```python
from build123d import *

# Parameters (mm, degrees)
SKETCH1_W           = 10
SKETCH1_H           = 27
BOSS_EXTRUDE1_DEPTH = 10
SKETCH2_R           = 2.5
CUT_EXTRUDE1_DEPTH  = 10
SKETCH3_W           = 4.7
SKETCH3_H           = 4.7
BOSS_EXTRUDE2_DEPTH = 40
SKETCH4_W           = 2
SKETCH4_H           = 62
CUT_EXTRUDE3_DEPTH  = 3
FILLET1_R           = 4
SKETCH5_R           = 3
CUT_EXTRUDE4_DEPTH  = 3
CUT_EXTRUDE5_DEPTH  = 3


with BuildPart() as part:
    # Sketch1 → Boss-Extrude1 (new body)
    with BuildSketch(Plane(origin=(0, 0, 0), x_dir=(1, 0, 0), z_dir=(0, 1, 0))):
        with Locations((0.146426278, 10.467599094)):
            Rectangle(SKETCH1_W, SKETCH1_H)
    extrude(amount=BOSS_EXTRUDE1_DEPTH)

    # Sketch2 → Cut-Extrude1 (cut)
    with BuildSketch(Plane(origin=(0, 10, 0), x_dir=(1, 0, 0), z_dir=(0, 1, 0))):
        with Locations(Location((0.146426278, 18.467599094, 0), (0, 0, 270))):
            Circle(SKETCH2_R)
        with Locations(Location((0.146426278, 10.467599094, 0), (0, 0, 270))):
            Circle(SKETCH2_R)
        with Locations(Location((0.146426278, 2.467599094, 0), (0, 0, 270))):
            Circle(SKETCH2_R)
    extrude(amount=-CUT_EXTRUDE1_DEPTH, mode=Mode.SUBTRACT)

    # Sketch3 → Boss-Extrude2 (add)
    with BuildSketch(Plane.XY.offset(3.032400906)):
        with Locations((0.146426278, 2.35)):
            Rectangle(SKETCH3_W, SKETCH3_H)
    extrude(amount=BOSS_EXTRUDE2_DEPTH)

    # Sketch4 → Cut-Extrude3 (cut)
    with BuildSketch(Plane(origin=(0, 0, 0), x_dir=(-1, 0, 0), z_dir=(0, -1, 0))):
        with Locations((-0.246426278, -12.032400906)):
            Rectangle(SKETCH4_W, SKETCH4_H)
    extrude(amount=-CUT_EXTRUDE3_DEPTH, mode=Mode.SUBTRACT)

    # Fillet1
    fillet1_edges = [part.edges().sort_by_distance(p)[0] for p in [
        (5.146426278, 5, 3.032400906),
        (-4.853573722, 5, 3.032400906),
        (-4.853573722, 5, -23.967599094),
        (5.146426278, 5, -23.967599094),
    ]]
    fillet(fillet1_edges, radius=FILLET1_R)

    # Sketch5 → Cut-Extrude4 (cut)
    with BuildSketch(Plane(origin=(0, 0, 0), x_dir=(-1, 0, 0), z_dir=(0, -1, 0))):
        with Locations((-0.146426278, 18.467599094)):
            Circle(SKETCH5_R)
        with Locations((-0.146426278, 10.467599094)):
            Circle(SKETCH5_R)
        with Locations((-0.146426278, 2.467599094)):
            Circle(SKETCH5_R)
    extrude(amount=-CUT_EXTRUDE4_DEPTH, mode=Mode.SUBTRACT)

    # Sketch6 → Cut-Extrude5 (cut)
    with BuildSketch(Plane(origin=(0, 0, 0), x_dir=(-1, 0, 0), z_dir=(0, -1, 0))):
        Polygon((-0.146426278, 18.467599094), (-0.146426278, 18.967599094), (4.853573722, 18.967599094), (4.853573722, 18.467599094), (4.853573722, 17.967599094), (-0.146426278, 17.967599094), align=None)
        Polygon((-0.146426278, 10.467599094), (-0.146426278, 10.967599094), (4.853573722, 10.967599094), (4.853573722, 10.467599094), (4.853573722, 9.967599094), (-0.146426278, 9.967599094), align=None)
        Polygon((-0.146426278, 2.467599094), (-0.146426278, 2.967599094), (4.853573722, 2.967599094), (4.853573722, 2.467599094), (4.853573722, 1.967599094), (-0.146426278, 1.967599094), align=None)
    extrude(amount=-CUT_EXTRUDE5_DEPTH, mode=Mode.SUBTRACT)


solid = part.part
```
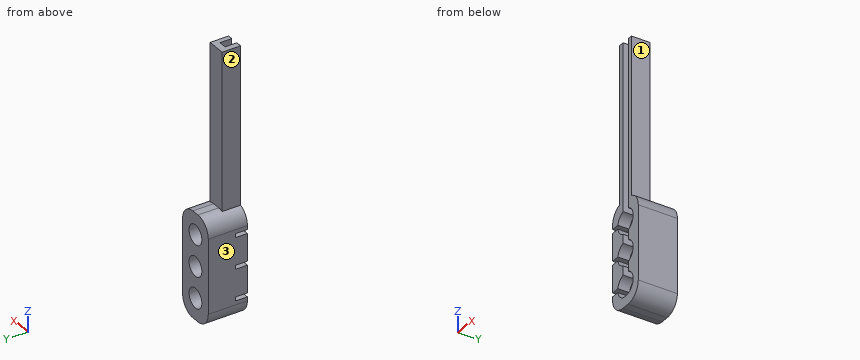
Geometry check sheet. Reference: the model listing, model coordinates, mm. Face numbers are marked on the shaded views. A direction names the side the tool comes from. Give positions to 0.01 mm unless a question says otherwise; leave off trailing zeros. Write each loop counter-clockwise with the first axis right and the second up, starting at its lowest first coordinate (ties: lowest second). Pieces come first, ordered by that corner, then holes.
1) Material ranges on L1, parallel to Z at x = 2.75, y = 2.5; L2, parallel to Z at x = -1.75, y = 9.5; L3, parallel to X at y = 8.75, z = -10.5, recorded low to high.
2) Section check D-D, the plane z = 4. Record the boundary of the cut face in (x, y), and give its area (3 significant figures).
3) Gauge pin test, flat ends, axial feed: pin 1 (1 mm diameter, centred on x = -3.5, y = 2, fed in from +Z); pin 2 (6 mm diameter, centred on y = 6, z = 5, fed in from +X); pin 3 (0.6 mm diameter, centred on x = -3.5, y = 1, fed in from -Z). Record the tip position at first contact, or that the pin passes through.
4) Access from +Z, -Z, +X, -X, +Y, -Y to the whole of each face (thin tool, end or side, straight path). Record for the marked faces 1, 2 and 3.
5) Section check A-A, the plane y = 1.5. State how many separate pieces and enclosed holes the cut face has, and give its area (3 significant figures).
6) Section check C-C, the plane z = -17. Record the boundary of the cut face in (x, y).
Computed:
1. L1: z = -23.63 to -19.96, -16.98 to -11.96, -8.98 to -3.96, -0.98 to 2.7
1. L2: z = -23.87 to -20.1, -16.84 to -12.1, -8.84 to -4.1, -0.84 to 2.93
1. L3: x = -4.85 to -2.35, 2.65 to 5.15
2. outline: (-2.2, 0) - (-0.75, 0) - (-0.75, 3) - (1.25, 3) - (1.25, 0) - (2.5, 0) - (2.5, 4.7) - (-2.2, 4.7) - close
2. area: 16.1 mm2
3. pin 1: stops at z = 2.41
3. pin 2: stops at x = 3.83
3. pin 3: stops at z = -23.21
4. face 1: +Z, +X, +Y, -Y
4. face 2: +Z, -X, +Y, -Y
4. face 3: +Z, -Z, -X, +Y, -Y
5. separate pieces: 4
5. enclosed holes: 0
5. area: 260 mm2
6. outline: (-4.85, 0) - (-2.47, 0) - (-2.47, 3) - (-1.88, 3) - (-1.88, 10) - (-4.85, 10) - close; (2.17, 3) - (2.76, 3) - (2.76, 0) - (5.15, 0) - (5.15, 10) - (2.17, 10) - close
